Study the drawing (mm; zero at the part's minimum x, y, z) and answer. Coordinates: 2 decimals unless noted, no trailing zeros. Loops run counter-clockwise (first coordinate to the right, second up) from the corner with the lowest first, then second, coordinate; pieces in that order, holes last. Notation, with made-up numbers: (-22, 6.25) - (19, 6.25) arc R18 cw to (19, 13.25) - close; hole circle Ø3 at (50, 80.25). An arc over 180 degrees is marked (long way). Use one line per item in the form item = value.
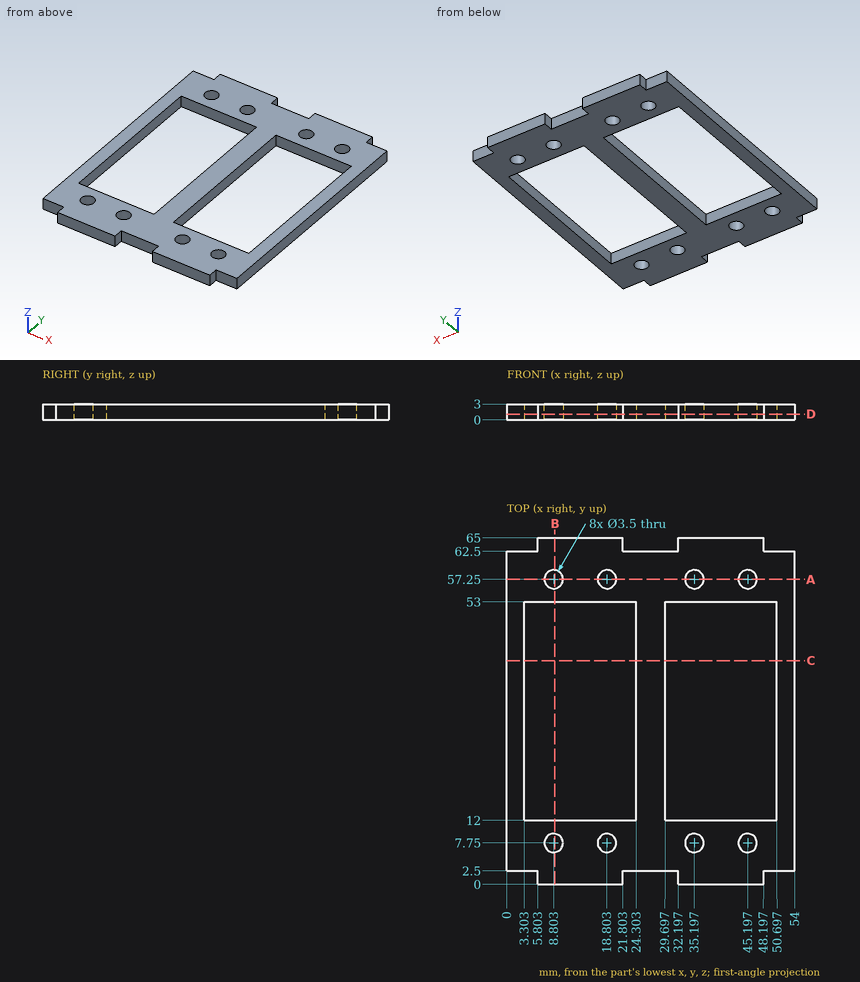
Item 1: The part is cut by section C-C on y = 42. Give the vertices of the cut face in (x, z).
Results below:
outline = (0, 0) - (3.3, 0) - (3.3, 3) - (0, 3) - close; (24.3, 0) - (29.7, 0) - (29.7, 3) - (24.3, 3) - close; (50.7, 0) - (54, 0) - (54, 3) - (50.7, 3) - close
Item 2: Each of these flat-tipped pins is pushed along its axis until it touches: P1, Ø4, axis at x = 8.8, y = 57.25, coming from the +Z side; P2, Ø1.2, axis at y = 63.5, z = 1.5, coming from the -X side; P3, Ø3, axis at x = 18.8, y = 7.75, coming from the -Z side; P4, Ø0.8, axis at y = 1, z = 2, coming from the +X side. Where does it stop, or does it pass through?
Results below:
P1 = 3
P2 = 5.8
P3 = through
P4 = 48.2
Item 3: Find the intervals of material crossed by L1, parallel to Y at x = 19, z = 2.8; L2, parallel to Y at x = 17, z = 1.6; L3, parallel to X at y = 46, z = 2.3, in increasing order.
Results below:
L1 = 0 to 6.01, 9.49 to 12, 53 to 55.51, 58.99 to 65
L2 = 0 to 12, 53 to 65
L3 = 0 to 3.3, 24.3 to 29.7, 50.7 to 54
Item 4: The part is cut by section A-A on y = 57.25. Give the vertices of the cut face in (x, z), plus the area to 3 significant figures.
Results below:
outline = (0, 0) - (7.05, 0) - (7.05, 3) - (0, 3) - close; (10.55, 0) - (17.05, 0) - (17.05, 3) - (10.55, 3) - close; (20.55, 0) - (33.45, 0) - (33.45, 3) - (20.55, 3) - close; (36.95, 0) - (43.45, 0) - (43.45, 3) - (36.95, 3) - close; (46.95, 0) - (54, 0) - (54, 3) - (46.95, 3) - close
area = 120 mm²
Item 5: The part is cut by section B-B on x = 9. Give the vertices of the cut face in (y, z).
Results below:
outline = (0, 0) - (6.01, 0) - (6.01, 3) - (0, 3) - close; (9.49, 0) - (12, 0) - (12, 3) - (9.49, 3) - close; (53, 0) - (55.51, 0) - (55.51, 3) - (53, 3) - close; (58.99, 0) - (65, 0) - (65, 3) - (58.99, 3) - close
Item 6: The part is cut by section D-D on z = 1.1. Count the separate pieces of the cut face and the enclosed holes in it, plus the area to 3 significant figures.
Results below:
separate_pieces = 1
enclosed_holes = 10
area = 1,600 mm²
